```python
from build123d import *

# Parameters (mm, degrees)
PAD_DEPTH       = 2
SKETCH001_W     = 50.25
SKETCH001_H     = 12
PAD001_DEPTH    = 10
POCKET_DEPTH    = 53.126
SKETCH003_W     = 15
SKETCH003_H     = 15
POCKET001_DEPTH = 0.5
PAD002_DEPTH    = 2
SKETCH005_R     = 1.2
POCKET002_DEPTH = 1.3
SKETCH006_R     = 2.25
POCKET003_DEPTH = 2.5
FILLET_R        = 1
FILLET001_R     = 0.5


with BuildPart() as part:
    # Sketch → Pad (new body)
    with BuildSketch(Plane.XY):
        with BuildLine():
            ThreePointArc((-28, 0), (0, -28), (28, 0))
            Line((28, 50), (28, 0))
            Line((-28, 50), (28, 50))
            Line((-28, 0), (-28, 50))
        make_face()
    extrude(amount=PAD_DEPTH)

    # Sketch001 → Pad001 (new body)
    with BuildSketch(Plane.XY.offset(2)):
        with Locations((0, 44)):
            Rectangle(SKETCH001_W, SKETCH001_H)
    extrude(amount=PAD001_DEPTH)

    # Sketch002 → Pocket (cut, through all)
    with BuildSketch(Plane.YZ.offset(25.125)):
        Polygon((50, 2), (47.399401, 9.281678), (39.394594, 6.422819), (39.058258, 7.36456), (34, 7.36456), (34, 14), (52, 14), (52, 2), align=None)
    extrude(amount=-POCKET_DEPTH, mode=Mode.SUBTRACT)

    # Sketch003 → Pocket001 (cut)
    with BuildSketch(Plane.XY.offset(2)):
        Rectangle(SKETCH003_W, SKETCH003_H)
    extrude(amount=-POCKET001_DEPTH, mode=Mode.SUBTRACT)

    # Sketch004 → Pad002 (new body)
    with BuildSketch(Plane.XY.offset(2)):
        with BuildLine():
            ThreePointArc((-25.125, 23.755002), (-18.625, 26.877501), (-25.125, 30))
            Line((-25.125, 30), (-25.125, 23.755002))
        make_face()
        with BuildLine():
            ThreePointArc((25.125, 30), (18.625, 26.877501), (25.125, 23.755002))
            Line((25.125, 30), (25.125, 23.755002))
        make_face()
        with BuildLine():
            ThreePointArc((3.283431, -24.90953), (0, -18.625), (-3.283431, -24.90953))
            ThreePointArc((-3.283431, -24.90953), (0, -25.125), (3.283431, -24.90953))
        make_face()
    extrude(amount=PAD002_DEPTH)

    # Sketch005 → Pocket002 (cut)
    with BuildSketch(Plane.XY.offset(4)):
        with Locations((-22.625, 26.8775)):
            Circle(SKETCH005_R)
        with Locations((22.625, 26.8775)):
            Circle(SKETCH005_R)
        with Locations((0, -22.625)):
            Circle(SKETCH005_R)
    extrude(amount=-POCKET002_DEPTH, mode=Mode.SUBTRACT)

    # Sketch006 → Pocket003 (cut)
    with BuildSketch(Plane(origin=(0, 0, 0), x_dir=(1, 0, 0), z_dir=(0, 0, -1))):
        with Locations((0, 22.625)):
            Circle(SKETCH006_R)
        with Locations((-22.625, -26.8775)):
            Circle(SKETCH006_R)
        with Locations((22.625, -26.8775)):
            Circle(SKETCH006_R)
    extrude(amount=-POCKET003_DEPTH, mode=Mode.SUBTRACT)

    # Fillet
    fillet_edges = [part.edges().sort_by_distance(p)[0] for p in [
        (-28, 50, 1),
        (28, 50, 1),
    ]]
    fillet(fillet_edges, radius=FILLET_R)

    # Fillet001
    fillet001_edges = [part.edges().sort_by_distance(p)[0] for p in [
        (0, 50, 0),
        (27.707107, 49.707107, 0),
        (28, 24.5, 0),
        (0, -28, 0),
        (-28, 24.5, 0),
        (-27.707107, 49.707107, 0),
    ]]
    fillet(fillet001_edges, radius=FILLET001_R)


solid = part.part
```
Here's how the part is built. I have some questions about the finished solid (model axes, mm). A direction names the side the tool comes from. Coordinates: 2 decimals unless noted, no trailing zeros. Order: outer loops, then holes, each group sorted by start corner. A loop starts at its lowest first (then second) coordinate and runs counter-clockwise, first axis right, second up. Notation, with made-up numbers: (61.25, 50.5) - (84.25, 50.5) arc R16 cw to (84.25, 69.5) - close; hole circle Ø5 at (13.5, 73). An arc over 180 degrees is marked (long way). One line per question, with ' | ' between items. Start each with the question number.
1. Which directions (+Z, -Z, +X, -X, +Y, -Y) give clear straight access to the entire face, cutting with the end or side of a thin tool? Please do faces 5 (the flat face through (25.125, 27, 3)), 6 (the cylindrical face through (-23.5, 27.7, 3.4)), 7 (the flat face through (-23, 27, 2.5)).
2. Please list where these lines run through material, in increasing order: line 1 along Y through (x, z) = (0, 1.45) (3 decimals); line 2 along Z through (x, y) = (-21, 4); line 3 along Z through (x, y) = (-21, 30). Write a range as [from, to].
3. If we mould it in two halves opening along X, with no side actions, what happens to faces 1 (the cylindrical face through (-0.046, -25.125, 2.986)), 2 (the cylindrical face through (-0.49, -20.43, 1.23)), 3 (the flat face through (0, -21, 4)), 4 (the flat face through (25.125, 44, 5))? For each: released by +X, released by -X, zero draft, split by the parting line, or undercut.
4. I'm going to push flat-ended pins straight in: pin 1 Ø2 at (x, y) = (-22.62, 26.88) entering from +Z; pin 2 Ø5 at (x, y) = (0, -22.625) entering from +Z; pin 3 Ø4 at (x, y) = (8.5, 26) entering from +Z. Where does each tip first touch, or does it pass through?
5. If we section it at A-A (x = 0): Write out the boundary of the cut face in (y, z) (3 decimals).
Model answer:
1) face 5: +Z, +X, +Y, -Y | face 6: +Z | face 7: -Z
2) line 1: y = [-28, -24.875], [-20.375, 50] | line 2: z = [0, 2] | line 3: z = [0, 4]
3) face 1: split by the parting line | face 2: undercut | face 3: zero draft | face 4: released by +X
4) pin 1: stops at z = 2.7 | pin 2: stops at z = 4 | pin 3: stops at z = 2
5) outline: (-28, 0.5) arc R0.5 ccw to (-27.5, 0) - (-24.875, 0) - (-24.875, 2.5) - (-20.375, 2.5) - (-20.375, 0) - (49.5, 0) arc R0.5 ccw to (50, 0.5) - (50, 2) - (47.399, 9.282) - (39.395, 6.423) - (39.058, 7.365) - (38, 7.365) - (38, 2) - (7.5, 2) - (7.5, 1.5) - (-7.5, 1.5) - (-7.5, 2) - (-18.625, 2) - (-18.625, 4) - (-21.425, 4) - (-21.425, 2.7) - (-23.825, 2.7) - (-23.825, 4) - (-25.125, 4) - (-25.125, 2) - (-28, 2) - close
